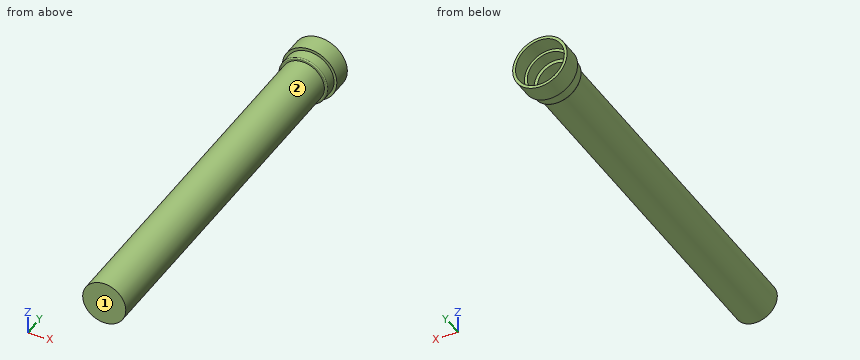
from build123d import *

# Parameters (mm, degrees)
FILLET2_R = 1


with BuildPart() as part:
    # Sketch1 → Revolve1 (revolve)
    with BuildSketch(Plane(origin=(0, 0, 0), x_dir=(0, 0, -1), z_dir=(1, 0, 0))):
        Polygon((-21.5, 0), (-24, 0), (-24, -17), (-21.5, -17), (-21.5, -28), (-19, -28), (-19, -350), (0, -350), (0, -347.5), (-16, -347.5), (-16, -345.435797774), (-16, -25.5), (-19, -25.5), (-19, -14.5), (-21.5, -14.5), align=None)
    revolve(axis=Axis((0, 0, 0), (0, -1, 0)))

    # Fillet2
    fillet2_edges = [part.edges().sort_by_distance(p)[0] for p in [
        (0, -28, -21.5),
    ]]
    fillet(fillet2_edges, radius=FILLET2_R)


solid = part.part
Build history of the part. All positions in model axes, mm. Face numbers are marked on the shaded views. A direction names the side the tool comes from. Round coordinates to 2 decimals unless told otherwise and drop trailing zeros. Order: outer loops, then holes, each group sorted by start corner. A loop starts at its lowest first (then second) coordinate and runs counter-clockwise, first axis right, second up. Notation, with made-up numbers: M 56.5,61 L 76.5,61 A19 ccw 76.5,75 Z; hole C -1,70 d3. An arc over 180 degrees is marked long. Use CSV: the item, a comma, the result in double quotes. Start each with the question number.
(1) Flat gauge pins, fed straight in: P1, Ø3, axis at y = -229.5, z = -10.5, coming from the +X side; P2, Ø2, axis at x = -2.5, z = 16.5, coming from the +Y side; P3, Ø5, axis at y = -273.5, z = 7.5, coming from the +X side. Where does each tip first touch, or does it go through?
(2) Tool access for the marked faces 1 and 2: list every direction of +Z, -Z, +X, -X, +Y, -Y with a clear straight run to the whole face (end or side of a thin tool).
(3) Cut at A-A on z = 0. List the corners of the cut face in (x, y), then the cut area to 3 significant figures.
(4) Cut at C-C on y = -62. List the corners of the cut face in (x, z).
(5) Drill centre lines: probe 1 along Z at (x, y) = (0, -20.75); probe 2 along X at (y, z) = (-11, 0). Where is each one in solid material? Low to high.
(6) Cut at B-B on x = 0. List the corners of the cut face in (y, z), then the cut area to 3 significant figures.
Findings:
1,P1,"stops at x = 16.73"
1,P2,"stops at y = -25.5"
1,P3,"stops at x = 18.33"
2,face 1,"+Z, -Z, +X, -X, -Y"
2,face 2,"-Y"
3,outline,"M -24,-17 L -21.5,-17 L -21.5,-27 A1 ccw -20.5,-28 L -19,-28 L -19,-350 L 19,-350 L 19,-28 L 20.5,-28 A1 ccw 21.5,-27 L 21.5,-17 L 24,-17 L 24,0 L 21.5,0 L 21.5,-14.5 L 19,-14.5 L 19,-25.5 L 16,-25.5 L 16,-347.5 L -16,-347.5 L -16,-25.5 L -19,-25.5 L -19,-14.5 L -21.5,-14.5 L -21.5,0 L -24,0 Z"
3,area,"2,180 mm^2"
4,outline,"C 0,0 d38; hole C 0,0 d32"
5,probe 1,"z = -21.5 to -19, 19 to 21.5"
5,probe 2,"x = -24 to -21.5, 21.5 to 24"
6,outline,"M -350,-19 L -28,-19 L -28,-20.5 A1 ccw -27,-21.5 L -17,-21.5 L -17,-24 L 0,-24 L 0,-21.5 L -14.5,-21.5 L -14.5,-19 L -25.5,-19 L -25.5,-16 L -347.5,-16 L -347.5,16 L -25.5,16 L -25.5,19 L -14.5,19 L -14.5,21.5 L 0,21.5 L 0,24 L -17,24 L -17,21.5 L -27,21.5 A1 ccw -28,20.5 L -28,19 L -350,19 Z"
6,area,"2,180 mm^2"
